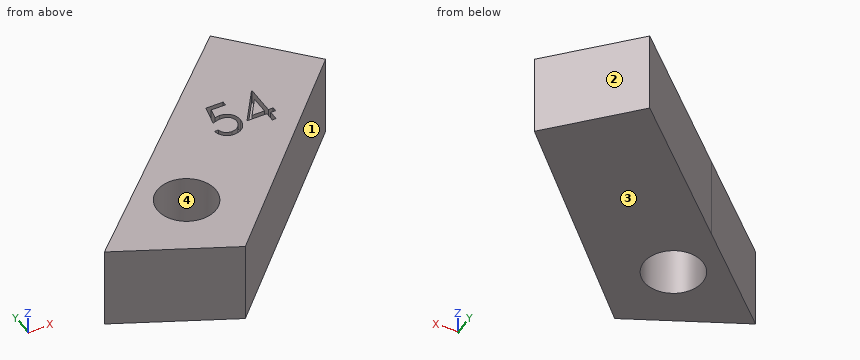
from build123d import *

# Parameters (mm, degrees)
SKETCH1_R           = 2.2
BOSS_EXTRUDE1_DEPTH = 6.2
CUT_EXTRUDE1_DEPTH  = 1


with BuildPart() as part:
    # Sketch1 → Boss-Extrude1 (new body)
    with BuildSketch(Plane(origin=(0, 0, 0), x_dir=(-1, 0, 0), z_dir=(0, 0, 1))):
        Polygon((-135.861235396, 102.40882942), (-149.806405315, 88.109421961), (-144.298520867, 82.333425686), (-134.435779681, 91.738355366), (-127.443880814, 98.405702296), align=None)
        with Locations((-134.779596853, 96.344682986)):
            Circle(SKETCH1_R, mode=Mode.SUBTRACT)
    extrude(amount=BOSS_EXTRUDE1_DEPTH)

    # Sketch2 → Cut-Extrude1 (cut)
    with BuildSketch(Plane.XY.offset(6.2)):
        with BuildLine():
            Line((141.757865871, -88.696242194), (141.757865871, -89.021883219))
            Line((141.757865871, -89.021883219), (140.677907938, -89.021883219))
            Line((140.677907938, -89.021883219), (140.506819196, -89.856974365))
            add(Edge.make_bspline(
                [(140.506819196, -89.856974365), (140.540434168, -89.847694047), (140.605557859, -89.829714899), (140.70167859, -89.809752521), (140.792930089, -89.797718869), (140.852144175, -89.796075751), (140.880797562, -89.795280655)],
                knots=[0, 0, 0, 0, 0.000104595, 0.000202637, 0.000294305, 0.000380252, 0.000380252, 0.000380252, 0.000380252], degree=3))
            add(Edge.make_bspline(
                [(140.880797562, -89.795280655), (140.916252097, -89.79604804), (140.985964572, -89.79755691), (141.087962759, -89.812045659), (141.185329027, -89.834851153), (141.277859748, -89.866710483), (141.365726105, -89.907450027), (141.448119678, -89.958340687), (141.526277214, -90.01778878), (141.598796567, -90.08613747), (141.664586475, -90.161359222), (141.722431337, -90.242238148), (141.771564544, -90.327988241), (141.811080372, -90.419428794), (141.842634732, -90.515548883), (141.863636899, -90.617359868), (141.877622056, -90.723902092), (141.879184507, -90.796749809), (141.879981255, -90.833897442)],
                knots=[0, 0, 0, 0, 0.000106308, 0.000209029, 0.000308378, 0.000405929, 0.000502102, 0.000598312, 0.00069588, 0.000796219, 0.000896736, 0.000995218, 0.001094066, 0.001192613, 0.001293582, 0.001396995, 0.001504047, 0.001615439, 0.001615439, 0.001615439, 0.001615439], degree=3))
            add(Edge.make_bspline(
                [(141.879981255, -90.833897442), (141.879377937, -90.859771171), (141.878179454, -90.911168967), (141.872084735, -90.987499777), (141.860350193, -91.062214633), (141.844595186, -91.135323445), (141.824145992, -91.206687805), (141.799390922, -91.276511976), (141.769095954, -91.34436137), (141.735866064, -91.410877978), (141.698449616, -91.474558052), (141.65692197, -91.534111061), (141.61304756, -91.590430374), (141.565838589, -91.642911975), (141.514856258, -91.691210998), (141.460718002, -91.735614082), (141.403855821, -91.776872146), (141.343389994, -91.813310437), (141.280667885, -91.846841119), (141.214783716, -91.874348899), (141.147237224, -91.898942021), (141.077056229, -91.91854495), (141.004399699, -91.933905196), (140.929147867, -91.944337883), (140.851695402, -91.951936509), (140.799194498, -91.952412175), (140.772674565, -91.95265245)],
                knots=[0, 0, 0, 0, 7.7636e-05, 0.000154223, 0.000229512, 0.000304362, 0.000378447, 0.000452077, 0.000526407, 0.000601214, 0.00067506, 0.000747747, 0.00081887, 0.000889121, 0.000959302, 0.001029336, 0.001099058, 0.00116985, 0.001240974, 0.00131221, 0.00138383, 0.001456517, 0.001530612, 0.001606437, 0.001684346, 0.001763871, 0.001763871, 0.001763871, 0.001763871], degree=3))
            add(Edge.make_bspline(
                [(140.772674565, -91.95265245), (140.741038701, -91.952025761), (140.678798876, -91.950792825), (140.587612361, -91.937894628), (140.499878398, -91.919421647), (140.416303235, -91.891630173), (140.336137874, -91.856807413), (140.260461551, -91.812796315), (140.187340597, -91.762922414), (140.119747535, -91.704066665), (140.057013061, -91.63973601), (140.000855014, -91.569924436), (139.950840983, -91.495784156), (139.907771884, -91.416955116), (139.871034394, -91.333644449), (139.842173654, -91.245540013), (139.818879718, -91.153102152), (139.809025044, -91.089462896), (139.804019717, -91.05713963)],
                knots=[0, 0, 0, 0, 9.4843e-05, 0.000186593, 0.000275792, 0.000363484, 0.000450342, 0.000537514, 0.000625728, 0.000715478, 0.000805885, 0.000894984, 0.00098389, 0.001073836, 0.001164117, 0.001256635, 0.001351658, 0.001449737, 0.001449737, 0.001449737, 0.001449737], degree=3))
            Line((139.804019717, -91.05713963), (140.088955614, -91.05713963))
            add(Edge.make_bspline(
                [(140.088955614, -91.05713963), (140.09596652, -91.08741684), (140.10944187, -91.14561132), (140.139019942, -91.227373322), (140.175183986, -91.300234332), (140.218186502, -91.365158169), (140.269485459, -91.421772045), (140.328022869, -91.472224665), (140.393652589, -91.517740675), (140.466580733, -91.5556799), (140.543518312, -91.588036555), (140.624042853, -91.609582735), (140.705961796, -91.624732831), (140.761368603, -91.626249357), (140.789211023, -91.627011425)],
                knots=[0, 0, 0, 0, 9.3172e-05, 0.000179081, 0.000260145, 0.000336703, 0.000411917, 0.000488562, 0.000568128, 0.000650923, 0.00073478, 0.000817953, 0.000900557, 0.000983994, 0.000983994, 0.000983994, 0.000983994], degree=3))
            add(Edge.make_bspline(
                [(140.789211023, -91.627011425), (140.816387612, -91.626266862), (140.869898538, -91.624800811), (140.948648867, -91.613516851), (141.024679117, -91.596138197), (141.097239077, -91.570130542), (141.167598473, -91.538521405), (141.233977536, -91.497958443), (141.298296575, -91.451276855), (141.358556382, -91.397794769), (141.413746454, -91.338857975), (141.462510935, -91.275832054), (141.503129992, -91.208597486), (141.53736022, -91.138318269), (141.563352855, -91.064224149), (141.581895745, -90.986662369), (141.592784234, -90.905441351), (141.59428209, -90.850042763), (141.595045358, -90.821813107)],
                knots=[0, 0, 0, 0, 8.15e-05, 0.000160473, 0.000238226, 0.000315066, 0.000391338, 0.000469218, 0.000547964, 0.000629516, 0.000710512, 0.000789892, 0.000868102, 0.000945761, 0.001024012, 0.00110315, 0.001184644, 0.001269321, 0.001269321, 0.001269321, 0.001269321], degree=3))
            add(Edge.make_bspline(
                [(141.595045358, -90.821813107), (141.594448023, -90.79634439), (141.593278825, -90.746492999), (141.583726093, -90.673559433), (141.567109983, -90.604550316), (141.544046892, -90.539132404), (141.514764767, -90.477243995), (141.478981326, -90.418821219), (141.43602503, -90.364634099), (141.386955959, -90.314657283), (141.333200451, -90.268533718), (141.273833627, -90.229214439), (141.210097836, -90.196136457), (141.142760985, -90.167590487), (141.070221399, -90.147088382), (140.993915596, -90.131696086), (140.913019583, -90.12279215), (140.857710459, -90.121556723), (140.829280134, -90.120921681)],
                knots=[0, 0, 0, 0, 7.6388e-05, 0.000149519, 0.000220172, 0.000288967, 0.000357247, 0.000425206, 0.000494043, 0.000564207, 0.000635056, 0.000706145, 0.000777268, 0.000850264, 0.000925136, 0.001002969, 0.001083601, 0.001168886, 0.001168886, 0.001168886, 0.001168886], degree=3))
            add(Edge.make_bspline(
                [(140.829280134, -90.120921681), (140.80467032, -90.12144836), (140.753857297, -90.122535819), (140.675913019, -90.130542712), (140.594005527, -90.143459787), (140.508448806, -90.161227311), (140.418985917, -90.184478359), (140.325805653, -90.212340799), (140.228712097, -90.245652898), (140.163291019, -90.270809978), (140.129660743, -90.283742194)],
                knots=[0, 0, 0, 0, 7.3822e-05, 0.000152423, 0.000234822, 0.000322511, 0.00041445, 0.000512043, 0.000614219, 0.000722306, 0.000722306, 0.000722306, 0.000722306], degree=3))
            Line((140.129660743, -90.283742194), (140.455301768, -88.696242194))
            Line((140.455301768, -88.696242194), (141.757865871, -88.696242194))
        make_face()
        Polygon((143.938770318, -88.614831937), (143.996647922, -88.614831937), (143.996647922, -90.81290886), (144.362994076, -90.81290886), (144.362994076, -91.138549886), (143.996647922, -91.138549886), (143.996647922, -91.871242194), (143.711712025, -91.871242194), (143.711712025, -91.138549886), (142.205622281, -91.138549886), align=None)
        Polygon((143.711712025, -90.81290886), (143.711712025, -89.434022643), (142.765317794, -90.81290886), align=None, mode=Mode.SUBTRACT)
    extrude(amount=-CUT_EXTRUDE1_DEPTH, mode=Mode.SUBTRACT)


solid = part.part
Geometry check sheet. Reference: the model listing, model coordinates, mm. Face numbers are marked on the shaded views. Give positions to 0.01 mm unless a question says otherwise; leave off trailing zeros. Write each loop counter-clockwise with the first axis right and the second up, starting at its lowest first coordinate (ties: lowest second). Pieces come first, ordered by that corner, then holes.
1) Cross-section at B-B (x = 135.5). Record the boundary of the cut face in (y, z).
Values follow:
outline: (-102.24, 0) - (-98.42, 0) - (-98.42, 6.2) - (-102.24, 6.2) - close; (-94.27, 0) - (-90.72, 0) - (-90.72, 6.2) - (-94.27, 6.2) - close
2) Cross-section at A-A (y = -95.5). Record the boundary of the cut face in (x, z), plus the area to 3 significant figures.
Values follow:
outline: (130.49, 0) - (132.75, 0) - (132.75, 6.2) - (130.49, 6.2) - close; (136.81, 0) - (142.6, 0) - (142.6, 6.2) - (136.81, 6.2) - close
area: 49.9 mm2
3) Cross-section at D-D (y = -93.25). Record the boundary of the cut face in (x, z), plus the area to 3 significant figures.
Values follow:
outline: (132.85, 0) - (144.79, 0) - (144.79, 6.2) - (132.85, 6.2) - close
area: 74.0 mm2
4) Cross-section at C-C (z = 5.5). Count the separate pieces of the cut face and the enclosed holes in it, plus the area to 3 significant figures.
Values follow:
separate pieces: 2
enclosed holes: 3
area: 162 mm2
5) Release check for a two-part mould opening along Y. For the marked faces 1, 2, 3 and 4 record: released by +Y, released by -Y, zero draft, split by the parting line, or undercut.
Values follow:
face 1: released by -Y
face 2: released by +Y
face 3: zero draft
face 4: undercut
6) Thickness scan on line 1 (X direction, y = -88.75, z = 5.75); line 2 (Y direction, x = 135.5, z = 1.25); line 3 (X direction, y = -95.5, z = 3). Record the ranges inside material, lowest first.
Values follow:
line 1: x = 137.57 to 140.44, 141.76 to 143.85, 144 to 149.18
line 2: y = -102.24 to -98.42, -94.27 to -90.72
line 3: x = 130.49 to 132.75, 136.81 to 142.6
7) Go/stop test with flat-tipped pins: pin 1 Ø0.5 at (x, z) = (141, 5.5) entering from -Y; pin 2 Ø3 at (x, z) = (143, 2) entering from -Y; pin 3 Ø0.5 at (x, z) = (143.5, 5.5) entering from +Y. Record where each tip stops, or that it passes through.
Values follow:
pin 1: stops at y = -97.4
pin 2: stops at y = -96.63
pin 3: stops at y = -82.86
